Source: three-view drawing plus pictorial views. Frame: mm from the lowest corner of the part. A direction names the side the tool comes from. Give positions to 0.01 mm unless a question says otherwise; leave off trailing zeros. Order: outer loops, then holes, each group sorted by start corner. A loop starts at its lowest first (then second) coordinate and runs counter-clockwise, first axis right, second up.
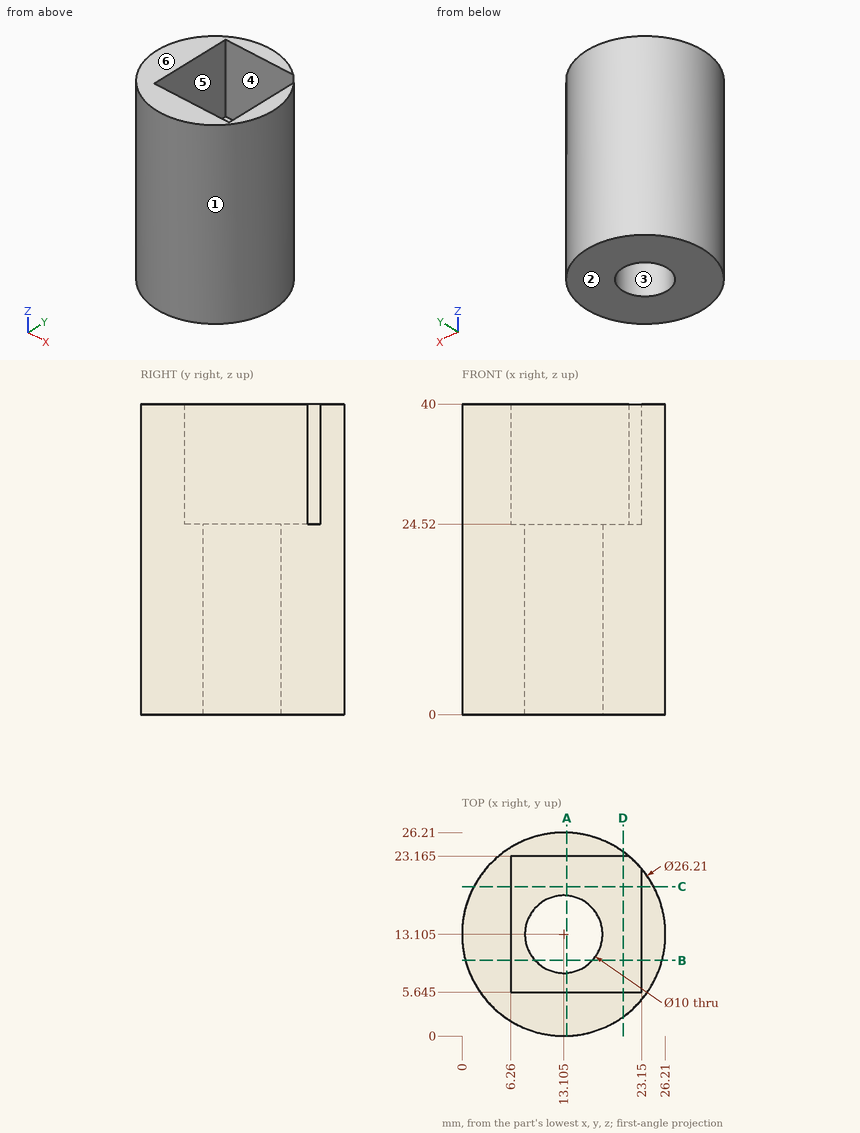
(1) Pin query (flat end, axial travel): pin 1 Ø3 at (x, z) = (6.5, 17.5) entering from -Y; pin 2 Ø2 at (x, z) = (23.5, 11) entering from -Y; pin 3 Ø11.5 at (x, y) = (13.105, 13.105) entering from +Z. Return the tip coordinate at first contact, or that it passes through.
(2) Section C-C, the plane y = 19.25. Return loops of the section in (x, z), plus the area to 3 significant figures.
(3) Draft query along X for the marked faces 1, 2 and 3. Return one class per face: +X half, -X half, draft (parallel to the pull), parting line (faces both ways), or undercut.
(4) Access query for the marked faces 4, 5 and 6. Directions: +Z, -Z, +X, -X, +Y, -Y. A direction counts if a zero-diameter tool reaches every point of the face in a straight line with its end or side. Return the directions, or none.
(5) Line query: line 1 along X through (y, z) = (13, 32); line 2 along Z through (x, y) = (20.75, 9.5); line 3 along Y through (x, z) = (8.5, 14). Output: solid intervals per line, ascending.
(6) Section B-B, the plane y = 9.75. Return loops of the section in (x, z).
(7) Section A-A, the plane x = 13.5. Return loops of the section in (y, z) (3 decimals).
(8) Section D-D, the plane x = 20.75. Return loops of the section in (y, z) (3 decimals), plus the area to 3 significant figures.
Checks:
1. pin 1: stops at y = 1.04
1. pin 2: stops at y = 3.97
1. pin 3: stops at z = 24.52
2. outline: (1.53, 0) - (24.68, 0) - (24.68, 40) - (23.15, 40) - (23.15, 24.52) - (6.26, 24.52) - (6.26, 40) - (1.53, 40) - close
2. area: 665 mm2
3. face 1: parting line
3. face 2: draft
3. face 3: undercut
4. face 4: +Z, +X
4. face 5: +Z
4. face 6: +Z, +X, -X, +Y, -Y
5. line 1: x = 0 to 6.26, 23.15 to 26.21
5. line 2: z = 0 to 24.52
5. line 3: y = 0.84 to 11.16, 15.05 to 25.37
6. outline: (0.44, 0) - (9.4, 0) - (9.4, 24.52) - (6.26, 24.52) - (6.26, 40) - (0.44, 40) - close; (16.81, 0) - (25.77, 0) - (25.77, 40) - (23.15, 40) - (23.15, 24.52) - (16.81, 24.52) - close
7. outline: (0.006, 0) - (8.121, 0) - (8.121, 24.52) - (5.645, 24.52) - (5.645, 40) - (0.006, 40) - close; (18.089, 0) - (26.204, 0) - (26.204, 40) - (23.165, 40) - (23.165, 24.52) - (18.089, 24.52) - close
8. outline: (2.461, 0) - (23.749, 0) - (23.749, 40) - (23.165, 40) - (23.165, 24.52) - (5.645, 24.52) - (5.645, 40) - (2.461, 40) - close
8. area: 580 mm2
